from build123d import *

# Parameters (mm, degrees)
SKETCH1_R           = 24
BOSS_EXTRUDE1_DEPTH = 2.3
SKETCH2_R           = 10
SKETCH2_R_2         = 3.5
CUT_EXTRUDE1_DEPTH  = 1.5
SKETCH3_R           = 20
SKETCH3_R_2         = 19
BOSS_EXTRUDE2_DEPTH = 1.6


with BuildPart() as part:
    # Sketch1 → Boss-Extrude1 (new body)
    with BuildSketch(Plane(origin=(0, 0, 0), x_dir=(1, 0, 0), z_dir=(0, 1, 0))):
        with Locations(Location((0, 0, 0), (0, 0, 270))):
            Circle(SKETCH1_R)
    extrude(amount=BOSS_EXTRUDE1_DEPTH)

    # Sketch2 → Cut-Extrude1 (cut)
    with BuildSketch(Plane(origin=(0, 2.3, 0), x_dir=(1, 0, 0), z_dir=(0, 1, 0))):
        with Locations(Location((0, 0, 0), (0, 0, 270))):
            Circle(SKETCH2_R)
        with Locations(Location((0, 0, 0), (0, 0, 270))):
            Circle(SKETCH2_R_2, mode=Mode.SUBTRACT)
    extrude(amount=-CUT_EXTRUDE1_DEPTH, mode=Mode.SUBTRACT)

    # Sketch3 → Boss-Extrude2 (add)
    with BuildSketch(Plane(origin=(0, 2.3, 0), x_dir=(1, 0, 0), z_dir=(0, 1, 0))):
        with Locations(Location((0, 0, 0), (0, 0, 270))):
            Circle(SKETCH3_R)
        with Locations(Location((0, 0, 0), (0, 0, 270))):
            Circle(SKETCH3_R_2, mode=Mode.SUBTRACT)
    extrude(amount=BOSS_EXTRUDE2_DEPTH)


solid = part.part
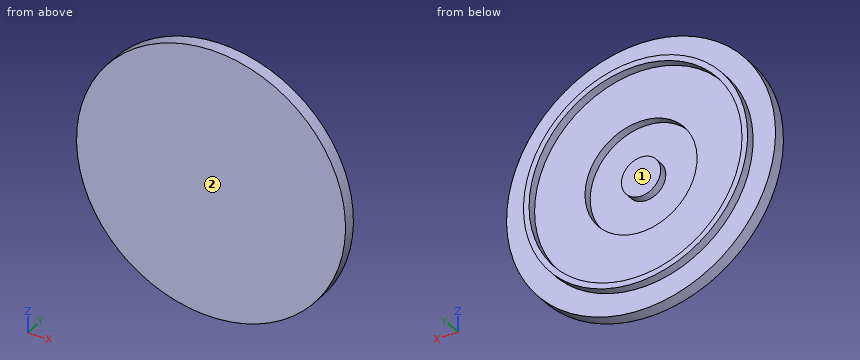
The listing builds one solid part. Answer for the finished solid, in the listing's coordinates (mm). Face numbers are marked on the shaded views. Round coordinates to 2 decimals unless told otherwise and drop trailing zeros. Write each loop counter-clockwise with the first axis right and the second up, starting at its lowest first coordinate (ties: lowest second). Pieces come first, ordered by that corner, then holes. Notation, with made-up numbers: M -18.5,22 L 34.5,22 A27 cw 34.5,47 Z; hole C -14.5,5 d2. An arc over 180 degrees is marked long. Write each question's results on one line, items separated by ' | '. Start each with the question number.
Item 1: A cutting plane is placed at A-A on y = 1.7. Write down the section's boundary in (x, z).
Item 2: Straight lines are drawn through the part: L1, parallel to X at y = 1.25, z = 0; L2, parallel to X at y = 2.7, z = 0; L3, parallel to X at y = 2.15, z = -2. For each, find the intervals that lie inside material, in ascending order. Write a range as [from, to].
Item 3: A cutting plane is placed at C-C on x = 0. Write down the section's boundary in (y, z).
Item 4: A cutting plane is placed at B-B on z = 0. Write down the section's boundary in (x, y), and give its area (3 significant figures).
Item 5: A flat-ended cylindrical pin translates along its axis: pin 1 Ø5.5 at (x, z) = (1.5, 0.5) entering from +Y. Find the tip coordinate at first contact, or state that the pin passes through.
Item 6: A cutting plane is placed at D-D on x = 8. Write down the section's boundary in (y, z), and give its area (3 significant figures).
Item 7: For a pull along Z with two mould halves and no side action, classify the marked faces 1 and 2 as pulls with the +Z half, pulls with the -Z half, needs draft (parallel to the pull), parting line crosses it, or undercut.
Check sheet entries:
1) outline: C 0,0 d48; C 0,0 d7; hole C 0,0 d20
2) L1: [-24, -10], [-3.5, 3.5], [10, 24] | L2: [-20, -19], [19, 20] | L3: [-23.92, -9.8], [-2.87, 2.87], [9.8, 23.92]
3) outline: M 0,-24 L 2.3,-24 L 2.3,-20 L 3.9,-20 L 3.9,-19 L 2.3,-19 L 2.3,-10 L 0.8,-10 L 0.8,-3.5 L 2.3,-3.5 L 2.3,3.5 L 0.8,3.5 L 0.8,10 L 2.3,10 L 2.3,19 L 3.9,19 L 3.9,20 L 2.3,20 L 2.3,24 L 0,24 Z
4) outline: M -24,0 L 24,0 L 24,2.3 L 20,2.3 L 20,3.9 L 19,3.9 L 19,2.3 L 10,2.3 L 10,0.8 L 3.5,0.8 L 3.5,2.3 L -3.5,2.3 L -3.5,0.8 L -10,0.8 L -10,2.3 L -19,2.3 L -19,3.9 L -20,3.9 L -20,2.3 L -24,2.3 Z | area: 94.1 mm²
5) pin 1: y = 2.3
6) outline: M 0,-22.63 L 2.3,-22.63 L 2.3,-18.33 L 3.9,-18.33 L 3.9,-17.23 L 2.3,-17.23 L 2.3,-6 L 0.8,-6 L 0.8,6 L 2.3,6 L 2.3,17.23 L 3.9,17.23 L 3.9,18.33 L 2.3,18.33 L 2.3,22.63 L 0,22.63 Z | area: 89.6 mm²
7) face 1: undercut | face 2: needs draft
